Input: part model. Units: mm. Frame: model coordinates. Face numbers are marked on the shaded views. A direction names the side the tool comes from. Coordinates: 2 decimals unless noted, no trailing zeros. Loops run counter-clockwise (first coordinate to the right, second up) from the corner with the lowest first, then second, coordinate; pieces in that order, holes last. Notation, with made-up numbers: (79, 67.5) - (137, 67.5) arc R21 cw to (137, 80.5) - close; hole circle Ø3 at (25.5, -34). An arc over 180 degrees is marked (long way). Write item = value, one per line. Start each with the question number.
from build123d import *

# Parameters (mm, degrees)
F0_R     = 4.35
F1_DEPTH = 2.35
F2_DEPTH = 1


with BuildPart() as f1:
    # F0 (on Front) → F1 (new body)
    with BuildSketch(Plane.XZ):
        with BuildLine():
            ThreePointArc((18.951979, 1.35), (18.987991, 0.675427), (19, 0))
            ThreePointArc((19, 0), (18.987991, -0.675427), (18.951979, -1.35))
            ThreePointArc((18.951979, -1.35), (13.435029, -13.435029), (1.35, -18.951979))
            ThreePointArc((1.35, -18.951979), (0, -19), (-1.35, -18.951979))
            ThreePointArc((-1.35, -18.951979), (-13.435029, -13.435029), (-18.951979, -1.35))
            ThreePointArc((-18.951979, -1.35), (-19, 0), (-18.951979, 1.35))
            ThreePointArc((-18.951979, 1.35), (-18.002767, 6.074569), (-15.895465, 10.408371))
            ThreePointArc((-15.895465, 10.408371), (-16.558319, 10.763563), (-17.163626, 11.209815))
            ThreePointArc((-17.163626, 11.209815), (-19.444888, 6.492022), (-20.4555, 1.35))
            ThreePointArc((-20.4555, 1.35), (-20.5, 0), (-20.4555, -1.35))
            ThreePointArc((-20.4555, -1.35), (-14.495689, -14.495689), (-1.35, -20.4555))
            ThreePointArc((-1.35, -20.4555), (0, -20.5), (1.35, -20.4555))
            ThreePointArc((1.35, -20.4555), (14.495689, -14.495689), (20.4555, -1.35))
            ThreePointArc((20.4555, -1.35), (20.488872, -0.675367), (20.5, 0))
            ThreePointArc((20.5, 0), (20.488872, 0.675367), (20.4555, 1.35))
            ThreePointArc((20.4555, 1.35), (14.495689, 14.495689), (1.35, 20.4555))
            ThreePointArc((1.35, 20.4555), (0, 20.5), (-1.35, 20.4555))
            ThreePointArc((-1.35, 20.4555), (-5.512738, 19.744866), (-9.441543, 18.196353))
            ThreePointArc((-9.441543, 18.196353), (-9.057906, 17.549546), (-8.770617, 16.854563))
            ThreePointArc((-8.770617, 16.854563), (-5.167834, 18.283695), (-1.35, 18.951979))
            ThreePointArc((-1.35, 18.951979), (0, 19), (1.35, 18.951979))
            ThreePointArc((1.35, 18.951979), (13.435029, 13.435029), (18.951979, 1.35))
        make_face()
        with BuildLine():
            ThreePointArc((5.95, 0), (5.911079, 0.679444), (5.794825, 1.35))
            ThreePointArc((5.794825, 1.35), (4.207285, 4.207285), (1.35, 5.794825))
            ThreePointArc((1.35, 5.794825), (0, 5.95), (-1.35, 5.794825))
            ThreePointArc((-1.35, 5.794825), (-4.207285, 4.207285), (-5.794825, 1.35))
            ThreePointArc((-5.794825, 1.35), (-5.95, 0), (-5.794825, -1.35))
            ThreePointArc((-5.794825, -1.35), (-4.207285, -4.207285), (-1.35, -5.794825))
            ThreePointArc((-1.35, -5.794825), (0, -5.95), (1.35, -5.794825))
            ThreePointArc((1.35, -5.794825), (4.207285, -4.207285), (5.794825, -1.35))
            ThreePointArc((5.794825, -1.35), (5.911079, -0.679444), (5.95, 0))
        make_face()
        Circle(F0_R, mode=Mode.SUBTRACT)
        with BuildLine():
            ThreePointArc((-18.951979, 1.35), (-19, 0), (-18.951979, -1.35))
            Line((-18.951979, -1.35), (-5.794825, -1.35))
            ThreePointArc((-5.794825, -1.35), (-5.95, 0), (-5.794825, 1.35))
            Line((-5.794825, 1.35), (-18.951979, 1.35))
        make_face()
        with BuildLine():
            Line((1.35, 5.794825), (1.35, 18.951979))
            ThreePointArc((1.35, 18.951979), (0, 19), (-1.35, 18.951979))
            Line((-1.35, 18.951979), (-1.35, 5.794825))
            ThreePointArc((-1.35, 5.794825), (0, 5.95), (1.35, 5.794825))
        make_face()
        with BuildLine():
            ThreePointArc((18.951979, -1.35), (18.987991, -0.675427), (19, 0))
            ThreePointArc((19, 0), (18.987991, 0.675427), (18.951979, 1.35))
            Line((18.951979, 1.35), (5.794825, 1.35))
            ThreePointArc((5.794825, 1.35), (5.911079, 0.679444), (5.95, 0))
            ThreePointArc((5.95, 0), (5.911079, -0.679444), (5.794825, -1.35))
            Line((5.794825, -1.35), (18.951979, -1.35))
        make_face()
        with BuildLine():
            ThreePointArc((-1.35, -18.951979), (0, -19), (1.35, -18.951979))
            Line((1.35, -18.951979), (1.35, -5.794825))
            ThreePointArc((1.35, -5.794825), (0, -5.95), (-1.35, -5.794825))
            Line((-1.35, -5.794825), (-1.35, -18.951979))
        make_face()
    extrude(amount=F1_DEPTH)

    # F0 (on Front) → F2 (join)
    with BuildSketch(Plane.XZ):
        with BuildLine():
            Line((-1.35, 5.794825), (-1.35, 18.951979))
            ThreePointArc((-1.35, 18.951979), (-5.167834, 18.283695), (-8.770617, 16.854563))
            ThreePointArc((-8.770617, 16.854563), (-10.231341, 11.308499), (-15.895465, 10.408371))
            ThreePointArc((-15.895465, 10.408371), (-18.002767, 6.074569), (-18.951979, 1.35))
            Line((-18.951979, 1.35), (-5.794825, 1.35))
            ThreePointArc((-5.794825, 1.35), (-4.207285, 4.207285), (-1.35, 5.794825))
        make_face()
        with BuildLine():
            Line((5.794825, 1.35), (18.951979, 1.35))
            ThreePointArc((18.951979, 1.35), (13.435029, 13.435029), (1.35, 18.951979))
            Line((1.35, 18.951979), (1.35, 5.794825))
            ThreePointArc((1.35, 5.794825), (4.207285, 4.207285), (5.794825, 1.35))
        make_face()
        with BuildLine():
            ThreePointArc((1.35, -18.951979), (13.435029, -13.435029), (18.951979, -1.35))
            Line((18.951979, -1.35), (5.794825, -1.35))
            ThreePointArc((5.794825, -1.35), (4.207285, -4.207285), (1.35, -5.794825))
            Line((1.35, -5.794825), (1.35, -18.951979))
        make_face()
        with BuildLine():
            ThreePointArc((-18.951979, -1.35), (-13.435029, -13.435029), (-1.35, -18.951979))
            Line((-1.35, -18.951979), (-1.35, -5.794825))
            ThreePointArc((-1.35, -5.794825), (-4.207285, -4.207285), (-5.794825, -1.35))
            Line((-5.794825, -1.35), (-18.951979, -1.35))
        make_face()
        with BuildLine():
            ThreePointArc((-20.4555, -1.35), (-20.5, 0), (-20.4555, 1.35))
            ThreePointArc((-20.4555, 1.35), (-21.8055, 0), (-20.4555, -1.35))
        make_face()
        with BuildLine():
            ThreePointArc((1.35, 20.4555), (0, 21.8055), (-1.35, 20.4555))
            ThreePointArc((-1.35, 20.4555), (0, 20.5), (1.35, 20.4555))
        make_face()
        with BuildLine():
            ThreePointArc((20.4555, -1.35), (21.8055, 0), (20.4555, 1.35))
            ThreePointArc((20.4555, 1.35), (20.488872, 0.675367), (20.5, 0))
            ThreePointArc((20.5, 0), (20.488872, -0.675367), (20.4555, -1.35))
        make_face()
        with BuildLine():
            ThreePointArc((1.35, -20.4555), (0, -20.5), (-1.35, -20.4555))
            ThreePointArc((-1.35, -20.4555), (0, -21.8055), (1.35, -20.4555))
        make_face()
    extrude(amount=F2_DEPTH)


solid = f1.part
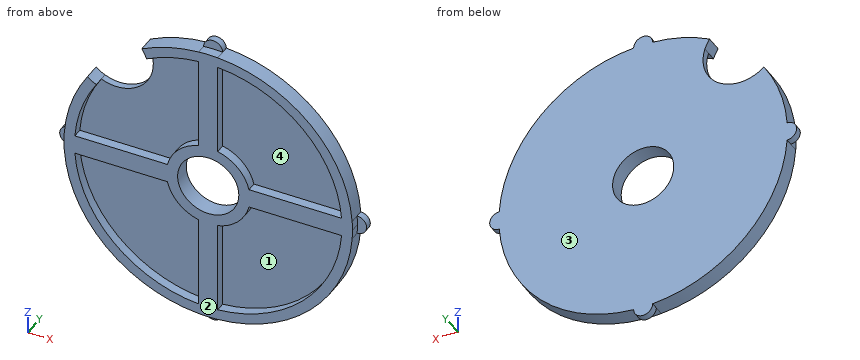
Item 1: Pin query (flat end, axial travel): pin 1 (0.7 mm diameter, centred on x = -21.5, z = -0.5, fed in from -Y); pin 2 (0.7 mm diameter, centred on x = 13, y = -2, fed in from +Z); pin 3 (1.1 mm diameter, centred on x = -14.5, y = -2, fed in from +Z); pin 4 (5.5 mm diameter, centred on x = 10, z = 13.5, fed in from -Y). Return the tip coordinate at first contact, or that it passes through.
Item 2: Access query for the marked faces 1 and 2. Directions: +Z, -Z, +X, -X, +Y, -Y. A direction counts if a zero-diameter tool reaches every point of the face in a straight line with its end or side. Return the directions, or none.
Item 3: Cut plane B-B on x = 0. Return loops of the section in (y, z).
Item 4: Cut plane C-C on z = -2. Return loops of the section in (x, y), plus the area to 3 significant figures.
Item 5: Cut plane A-A on y = -0.6. Return loops of the section in (x, z).
Item 6: Ray query, line 1 (Z direction, x = 0, y = -1.35); line 2 (Z direction, x = 0, y = -0.9); line 3 (X direction, y = -1.9, z = 10). Return the intervals inside material, ascending.
Item 7: Cut plane D-D on z = 8. Return loops of the section in (x, y), plus the area to 3 significant figures.
Item 8: Pull-direction query (X, two-part tool) for the marked faces 3 and 4; classes: pulls with the +X half, pulls with the -X half, needs draft (parallel to the pull), parting line crosses it, or undercut.
Recorded:
q1.pin_1 = -1
q1.pin_2 = 16.13
q1.pin_3 = 1.35
q1.pin_4 = -2.35
q2.face_1 = -Y
q2.face_2 = +Z, -Z, +X, -X, -Y
q3.outline = (-2.35, -20.5) - (-1, -20.5) - (-1, -21.81) - (0, -21.81) - (0, -4.35) - (-2.35, -4.35) - close; (-2.35, 4.35) - (0, 4.35) - (0, 21.81) - (-1, 21.81) - (-1, 20.5) - (-2.35, 20.5) - close
q4.outline = (-20.4, -2.35) - (-18.89, -2.35) - (-18.89, -1) - (-5.6, -1) - (-5.6, -2.35) - (-3.86, -2.35) - (-3.86, 0) - (-20.4, 0) - close; (3.86, -2.35) - (5.6, -2.35) - (5.6, -1) - (18.89, -1) - (18.89, -2.35) - (20.4, -2.35) - (20.4, 0) - (3.86, 0) - close
q4.area = 41.8 mm²
q5.outline = (-20.46, -1.35) arc R20.5 ccw to (-1.35, -20.46) arc R1.35 ccw to (1.35, -20.46) arc R20.5 ccw to (20.46, -1.35) arc R1.35 ccw to (20.46, 1.35) arc R20.5 ccw to (1.35, 20.46) arc R1.35 ccw to (-1.35, 20.46) arc R20.5 ccw to (-9.44, 18.2) arc R5.25 cw to (-8.77, 16.85) arc R5.25 cw to (-15.9, 10.41) arc R5.25 cw to (-17.16, 11.21) arc R20.5 ccw to (-20.46, 1.35) arc R1.35 ccw to start; hole circle Ø8.7 at (0, 0)
q6.line_1 = -20.5 to -4.35, 4.35 to 20.5
q6.line_2 = -21.81 to -4.35, 4.35 to 21.81
q6.line_3 = -17.9 to -16.16, -1.35 to 1.35, 16.16 to 17.9
q7.outline = (-18.87, -2.35) - (-17.23, -2.35) - (-17.23, -1) - (-1.35, -1) - (-1.35, -2.35) - (1.35, -2.35) - (1.35, -1) - (17.23, -1) - (17.23, -2.35) - (18.87, -2.35) - (18.87, 0) - (-18.87, 0) - close
q7.area = 45.8 mm²
q8.face_3 = needs draft
q8.face_4 = undercut
